from build123d import *

# Parameters (mm, degrees)
ESQUISSE1_R             = 13
BOSS_EXTRU_1_DEPTH      = 6
ESQUISSE2_R             = 1.5
ENL_V_MAT_EXTRU_1_DEPTH = 10


with BuildPart() as part:
    # Esquisse1 → Boss.-Extru.1 (new body)
    with BuildSketch(Plane.XY):
        Polygon((41.794604007, 40), (60, 14), (60, 0), (0, 0), (0, 14), (18.205395993, 40), align=None)
        with Locations((30, 14)):
            Circle(ESQUISSE1_R, mode=Mode.SUBTRACT)
    extrude(amount=BOSS_EXTRU_1_DEPTH)

    # Esquisse2 → Enlèv. mat.-Extru.1 (cut)
    with BuildSketch(Plane.XY.offset(6)):
        with Locations((16.252272915, 4)):
            Circle(ESQUISSE2_R)
        with Locations((43.747727085, 4)):
            Circle(ESQUISSE2_R)
        with Locations((30, 31)):
            Circle(ESQUISSE2_R)
    extrude(amount=-ENL_V_MAT_EXTRU_1_DEPTH, mode=Mode.SUBTRACT)


solid = part.part
The model under review builds one solid part; all positions refer to its coordinate system, in mm. Round coordinates to 2 decimals unless told otherwise and drop trailing zeros. Loops run counter-clockwise (first coordinate to the right, second up) from the corner with the lowest first, then second, coordinate; pieces in that order, holes last. Notation, with made-up numbers: (-20, -29) -> (-15, -29) arc R35 ccw to (-15, 6) -> close; hole circle Ø6 at (56, -29.75). An arc over 180 degrees is marked (long way). One line per question, with ' | ' between items. Start each with the question number.
Item 1: Wall thickness on line 1 along Y through (x, z) = (30, 1.8); line 2 along Y through (x, z) = (40.5, 0.4); line 3 along Y through (x, z) = (28, 0.7): over which ranges is each line inside the solid? List them lowest first. Write a range as [from, to].
Item 2: Add section B-B, the plane x = 30. Write out the cut boundary in (y, z), then the cut area to 3 significant figures.
Item 3: Add section C-C, the plane y = 31. Write out the cut boundary in (x, z).
Item 4: Add section A-A, the plane z = 3.45. Write out the cut boundary in (x, y), then the cut area to 3 significant figures.
Item 5: Draft analysis for pull direction X (two halves, no side actions). For faces 1 (the face through (19.684, 6.09, 2.958)), 2 (the face through (30, 29, 6)), 3 (the face through (60, 7, 3)), state which applies: +X half, -X half, draft (parallel to the pull), parting line (faces both ways), or undercut.
Item 6: Add section D-D, the plane x = 39.5. Write out the cut boundary in (y, z).
Return value:
1) line 1: y = [0, 1], [27, 29.5], [32.5, 40] | line 2: y = [0, 6.34], [21.66, 40] | line 3: y = [0, 1.15], [26.85, 40]
2) outline: (0, 0) -> (1, 0) -> (1, 6) -> (0, 6) -> close; (27, 0) -> (29.5, 0) -> (29.5, 6) -> (27, 6) -> close; (32.5, 0) -> (40, 0) -> (40, 6) -> (32.5, 6) -> close | area: 66.0 mm2
3) outline: (11.9, 0) -> (28.5, 0) -> (28.5, 6) -> (11.9, 6) -> close; (31.5, 0) -> (48.1, 0) -> (48.1, 6) -> (31.5, 6) -> close
4) outline: (0, 0) -> (60, 0) -> (60, 14) -> (41.79, 40) -> (18.21, 40) -> (0, 14) -> close; hole circle Ø3 at (16.25, 4); hole circle Ø26 at (30, 14); hole circle Ø3 at (30, 31); hole circle Ø3 at (43.75, 4) | area: 1,370 mm2
5) face 1: undercut | face 2: draft | face 3: +X half
6) outline: (0, 0) -> (5.13, 0) -> (5.13, 6) -> (0, 6) -> close; (22.87, 0) -> (40, 0) -> (40, 6) -> (22.87, 6) -> close
